from build123d import *

# Parameters (mm, degrees)
SKETCH1_R                  = 43
BOSS_EXTRUDE1_DEPTH        = 0.75
F_3_2_3_2_DIAMETER_HOLE1_D = 3.2
CUT_EXTRUDE1_DEPTH         = 2.5


with BuildPart() as part:
    # Sketch1 → Boss-Extrude1 (new body, symmetric)
    with BuildSketch(Plane(origin=(0, 0, 0), x_dir=(1, 0, 0), z_dir=(0, 1, 0))):
        Circle(SKETCH1_R)
    extrude(amount=BOSS_EXTRUDE1_DEPTH, both=True)

    # Ø3.2 (3.2) Diameter Hole1 (through all)
    with Locations(Plane(origin=(0, 0.75, 0), x_dir=(1, 0, 0), z_dir=(0, 1, 0))):
        with Locations((-34.208003449, 19.75), (-34.208003449, -19.75), (-31.112698372, 0), (19.75, 34.208003449), (-19.75, 34.208003449), (0, 31.112698372), (34.208003449, -19.75), (34.208003449, 19.75), (31.112698372, 0), (-19.75, -34.208003449), (19.75, -34.208003449), (0, -31.112698372), (0, 0)):
            Hole(F_3_2_3_2_DIAMETER_HOLE1_D / 2)

    # Sketch4 → Cut-Extrude1 (cut, through all)
    with BuildSketch(Plane(origin=(0, 0.75, 0), x_dir=(1, 0, 0), z_dir=(0, 1, 0))):
        with BuildLine():
            ThreePointArc((-35.627121412, -5.167999605), (-25.455844123, -25.455844123), (-5.167999605, -35.627121412))
            ThreePointArc((-5.167999605, -35.627121412), (-3.250695933, -34.80648789), (-3.106019964, -32.725968337))
            ThreePointArc((-3.106019964, -32.725968337), (0, -27.612698372), (3.106019964, -32.725968337))
            ThreePointArc((3.106019964, -32.725968337), (3.250695933, -34.80648789), (5.167999605, -35.627121412))
            ThreePointArc((5.167999605, -35.627121412), (25.455844123, -25.455844123), (35.627121412, -5.167999605))
            ThreePointArc((35.627121412, -5.167999605), (34.80648789, -3.250695933), (32.725968337, -3.106019964))
            ThreePointArc((32.725968337, -3.106019964), (27.612698372, 0), (32.725968337, 3.106019964))
            ThreePointArc((32.725968337, 3.106019964), (34.80648789, 3.250695933), (35.627121412, 5.167999605))
            ThreePointArc((35.627121412, 5.167999605), (25.455844123, 25.455844123), (5.167999605, 35.627121412))
            ThreePointArc((5.167999605, 35.627121412), (3.250695933, 34.80648789), (3.106019964, 32.725968337))
            ThreePointArc((3.106019964, 32.725968337), (0, 27.612698372), (-3.106019964, 32.725968337))
            ThreePointArc((-3.106019964, 32.725968337), (-3.250695933, 34.80648789), (-5.167999605, 35.627121412))
            ThreePointArc((-5.167999605, 35.627121412), (-25.455844123, 25.455844123), (-35.627121412, 5.167999605))
            ThreePointArc((-35.627121412, 5.167999605), (-34.80648789, 3.250695933), (-32.725968337, 3.106019964))
            ThreePointArc((-32.725968337, 3.106019964), (-27.612698372, 0), (-32.725968337, -3.106019964))
            ThreePointArc((-32.725968337, -3.106019964), (-34.80648789, -3.250695933), (-35.627121412, -5.167999605))
        make_face()
    extrude(amount=-CUT_EXTRUDE1_DEPTH, mode=Mode.SUBTRACT)


solid = part.part
Can you work these out from the model? Positions are in its coordinate system, mm. Coordinates: 2 decimals unless noted, no trailing zeros. Write each loop counter-clockwise with the first axis right and the second up, starting at its lowest first coordinate (ties: lowest second). Pieces come first, ordered by that corner, then holes. Notation, with made-up numbers: (82, 35.5) - (124, 35.5) arc R17 cw to (124, 43.5) - close; hole circle Ø11 at (76, -7). An arc over 180 degrees is marked (long way). Return JSON: item names as keys, results as strings. Group by question number.
Item 1: If we section it at A-A (x = 0): Write out the boundary of the cut face in (y, z).
Item 2: If we section it at D-D (x = 12.5): Write out the boundary of the cut face in (y, z), then the cut area to 3 significant figures.
Item 3: If we section it at C-C (z = 0): Write out the boundary of the cut face in (x, y).
Item 4: We'd pull the mould along X, two halves only. Please class faces 1 (the face through (25.68, 0.01, -25.23)), 2 (the face through (-5.598, 0.01, -42.634)): pulls with the +X half, pulls with the -X half, needs draft (parallel to the pull), parting line crosses it, or undercut.
Item 5: If we section it at B-B (z = -24.5): Write out the boundary of the cut face in (x, y), then the cut area to 3 significant figures.
Item 6: Please list where these lines run through material, in increasing order: probe 1 along Z at (x, y) = (0, -0.35); probe 2 along X at (y, z) = (-0.2, -19.75).
Return value:
{
 "1": {"outline": "(-0.75, -43) - (0.75, -43) - (0.75, -32.71) - (-0.75, -32.71) - close; (-0.75, -29.51) - (0.75, -29.51) - (0.75, -27.61) - (-0.75, -27.61) - close; (-0.75, 27.61) - (0.75, 27.61) - (0.75, 29.51) - (-0.75, 29.51) - close; (-0.75, 32.71) - (0.75, 32.71) - (0.75, 43) - (-0.75, 43) - close"},
 "2": {"outline": "(-0.75, -41.14) - (0.75, -41.14) - (0.75, -33.76) - (-0.75, -33.76) - close; (-0.75, 33.76) - (0.75, 33.76) - (0.75, 41.14) - (-0.75, 41.14) - close", "area": "22.1 mm^2"},
 "3": {"outline": "(-43, -0.75) - (-32.71, -0.75) - (-32.71, 0.75) - (-43, 0.75) - close; (-29.51, -0.75) - (-27.61, -0.75) - (-27.61, 0.75) - (-29.51, 0.75) - close; (27.61, -0.75) - (29.51, -0.75) - (29.51, 0.75) - (27.61, 0.75) - close; (32.71, -0.75) - (43, -0.75) - (43, 0.75) - (32.71, 0.75) - close"},
 "4": {"face 1": "undercut", "face 2": "parting line crosses it"},
 "5": {"outline": "(-35.34, -0.75) - (-26.38, -0.75) - (-26.38, 0.75) - (-35.34, 0.75) - close; (26.38, -0.75) - (35.34, -0.75) - (35.34, 0.75) - (26.38, 0.75) - close", "area": "26.9 mm^2"},
 "6": {"probe 1": "z = -43 to -32.71, -29.51 to -27.61, 27.61 to 29.51, 32.71 to 43", "probe 2": "x = -38.2 to -35.81, -32.61 to -30.1, 30.1 to 32.61, 35.81 to 38.2"}
}
